```python
from build123d import *

# Parameters (mm, degrees)
F0_R     = 11.125
F0_R_2   = 4
F1_DEPTH = 3.5
F2_R     = 9.625
F2_R_2   = 5.5
F3_DEPTH = 12.5
F4_DEPTH = 3


with BuildPart() as f1:
    # F0 (on Top) → F1 (new body, symmetric)
    with BuildSketch(Plane.XY):
        Circle(F0_R)
        Circle(F0_R_2, mode=Mode.SUBTRACT)
    extrude(amount=F1_DEPTH, both=True)

    # F2 (on Top) → F3 (cut, symmetric)
    with BuildSketch(Plane.XY):
        Circle(F2_R)
        Circle(F2_R_2, mode=Mode.SUBTRACT)
    extrude(amount=F3_DEPTH, both=True, mode=Mode.SUBTRACT)

    # F2 (on Top) → F4 (join, symmetric)
    with BuildSketch(Plane.XY):
        Circle(F2_R)
        Circle(F2_R_2, mode=Mode.SUBTRACT)
    extrude(amount=F4_DEPTH, both=True)


solid = f1.part
```
The model under review builds one solid part; all positions refer to its coordinate system, in mm. A direction names the side the tool comes from. Round coordinates to 2 decimals unless told otherwise and drop trailing zeros. Order: outer loops, then holes, each group sorted by start corner. A loop starts at its lowest first (then second) coordinate and runs counter-clockwise, first axis right, second up.
(1) Take a section at D-D, the plane z = 2.5. State the section outline as (x, y) points (3 decimals).
Working result:
outline: circle Ø22.25 at (0, 0); hole circle Ø8 at (0, 0)
(2) Wall thickness on L1, parallel to Y at x = 0, z = 3.2 (3 decimals); L2, parallel to Y at x = 0, z = 2 (3 decimals); L3, parallel to X at y = -2.75, z = -1: over which ranges is each line inside the solid? List them lowest first.
Working result:
L1: y = -11.125 to -9.625, -5.5 to -4, 4 to 5.5, 9.625 to 11.125
L2: y = -11.125 to -4, 4 to 11.125
L3: x = -10.78 to -2.9, 2.9 to 10.78
(3) For P1, Ø4, axis at x = 8.5, z = 1.5, coming from the +Y side; P2, Ø7, axis at x = 0, y = 0, coming from the -Z side; P3, Ø3, axis at x = 3, z = 1, coming from the -Y side, all flat-tipped, find the tip position at first contact; note any pin that passes through.
Working result:
P1: stops at y = 9.03
P2: passes through
P3: stops at y = -11.02
(4) Take a section at C-C, the plane x = 8.5. State the section outline as (y, z) points, plus the area to 3 significant figures.
Working result:
outline: (-7.18, -3.5) - (-4.52, -3.5) - (-4.52, -3) - (4.52, -3) - (4.52, -3.5) - (7.18, -3.5) - (7.18, 3.5) - (4.52, 3.5) - (4.52, 3) - (-4.52, 3) - (-4.52, 3.5) - (-7.18, 3.5) - close
area: 91.5 mm2
(5) Take a section at A-A, the plane y = 0. State the section outline as (x, z) points (3 decimals).
Working result:
outline: (-11.125, -3.5) - (-9.625, -3.5) - (-9.625, -3) - (-5.5, -3) - (-5.5, -3.5) - (-4, -3.5) - (-4, 3.5) - (-5.5, 3.5) - (-5.5, 3) - (-9.625, 3) - (-9.625, 3.5) - (-11.125, 3.5) - close; (4, -3.5) - (5.5, -3.5) - (5.5, -3) - (9.625, -3) - (9.625, -3.5) - (11.125, -3.5) - (11.125, 3.5) - (9.625, 3.5) - (9.625, 3) - (5.5, 3) - (5.5, 3.5) - (4, 3.5) - close
(6) Mouldability with a two-part tool opening along Y and no side actions: class faces 4 (the face through (-7.638, -5.857, -3.246)), 5 (the face through (-8.2, 7.52, 0.05)), 6 (the face through (-4, -2, 3.5)) as released by +Y, released by -Y, zero draft, split by the parting line, or undercut.
Working result:
face 4: undercut
face 5: split by the parting line
face 6: zero draft
(7) Tool access review of faces 1 (the face through (-0.867, -3.905, -0.049)), 2 (the face through (-1.19, -5.37, -3.25)), 3 (the face through (4, -4, 3)): name each direction out of +Z, -Z, +X, -X, +Y, -Y from which nothing blocks a thin tool from reaching the whole face with its end or side.
Working result:
face 1: +Z, -Z
face 2: -Z
face 3: +Z
